from build123d import *

# Parameters (mm, degrees)
F1_DEPTH = 6.35
F2_SIZE  = 6.34999
F3_SIZE2 = 6.0462521685
F3_SIZE  = 34.29


# Not quite as in the source:
# - a fillet or chamfer is up to 0.001 mm smaller than in the source, because OpenCascade refuses the exact size


with BuildPart() as f1:
    # F0 (on Top) → F1 (new body)
    with BuildSketch(Plane.XY):
        Polygon((75, -225), (75, 225), (29.020415619, 152.489066124), (29.020415619, -152.489066124), align=None)
    extrude(amount=F1_DEPTH)

    # F2 (size 6.35 in the source; OpenCascade refuses exactly that, so slightly less here)
    f2_edges = [f1.edges().sort_by_distance(p)[0] for p in [
        (75, 0, 0),
    ]]
    chamfer(f2_edges, length=F2_SIZE)

    # F3
    f3_edges = [f1.edges().sort_by_distance(p)[0] for p in [
        (29.020416, 0, 6.35),
    ]]
    f3_side = f1.faces().sort_by_distance((53.482225, 0, 6.35))[0]
    chamfer(f3_edges, length=F3_SIZE, length2=F3_SIZE2, reference=f3_side)


solid = f1.part
Build history of the part. All positions in model axes, mm. Coordinates: 2 decimals unless noted, no trailing zeros. Order: outer loops, then holes, each group sorted by start corner. A loop starts at its lowest first (then second) coordinate and runs counter-clockwise, first axis right, second up. Notation, with made-up numbers: M 54,2.5 L 89,2.5 A18 cw 89,34.5 Z; hole C 54,-20 d3. An arc over 180 degrees is marked long. One line per question, with ' | ' between items. Start each with the question number.
Q1. Probe L1, parallel to Z at x = 63, y = 113; L2, parallel to Z at x = 72, y = -183; L3, parallel to Y at x = 56, z = 5. List the from-to ranges inside material, lowest first. Write a range as from..to.
Q2. Saw through at C-C (x = 33.5). List the corners of the cut face in (y, z).
Q3. Flat gauge pin, fed straight in: pin 1 Ø5 at (x, y) = (49.5, -113) entering from +Z. Where does the tip first touch, or does it go through?
Q4. Saw through at B-B (z = 3.25). List the corners of the cut face in (x, y), then the cut area to 3 significant figures.
Check values:
1) L1: z = 0..6.3 | L2: z = 3.35..6.35 | L3: y = -195.04..195.04
2) outline: M -159.55,0 L 159.55,0 L 159.55,1.09 L -159.55,1.09 Z
3) pin 1: stops at z = 4.36
4) outline: M 45.73,-178.84 L 71.9,-220.11 L 71.9,220.11 L 45.73,178.84 Z | area: 10,400 mm2
